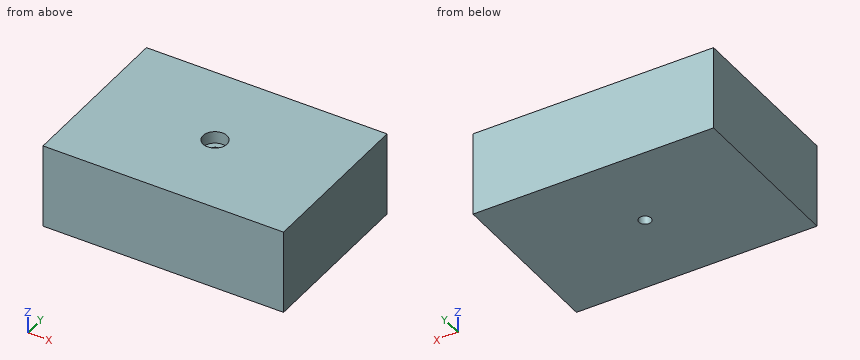
```python
from build123d import *

# Parameters (mm, degrees)
F0_W           = 100
F0_H           = 70
F1_DEPTH       = 17.5
F4_D           = 5
F4_CBORE_D     = 10
F4_CBORE_DEPTH = 5


with BuildPart() as f1:
    # F0 (on Top) → F1 (new body, symmetric)
    with BuildSketch(Plane.XY):
        Rectangle(F0_W, F0_H)
    extrude(amount=F1_DEPTH, both=True)

    # F4 (through all)
    with Locations(Plane.XY.offset(17.5)):
        with Locations((0, 0)):
            CounterBoreHole(F4_D / 2, F4_CBORE_D / 2, F4_CBORE_DEPTH)


solid = f1.part
```
The listing builds one solid part. Answer for the finished solid, in the listing's coordinates (mm). Coordinates: 2 decimals unless noted, no trailing zeros. Loops run counter-clockwise (first coordinate to the right, second up) from the corner with the lowest first, then second, coordinate; pieces in that order, holes last. Notation, with made-up numbers: (53, 88) -> (81, 88) arc R30 ccw to (81, 110) -> close; hole circle Ø5 at (47, -3.75). An arc over 180 degrees is marked (long way). Use one line per item in the form item = value. Start each with the question number.
Item 1: A flat-ended cylindrical pin translates along its axis: pin 1 Ø3 at (x, y) = (-2, 2) entering from +Z. Find the tip coordinate at first contact, or state that the pin passes through.
Item 2: Consider L1, parallel to Y at x = 0, z = 4; L2, parallel to Y at x = 0, z = 14.2; L3, parallel to X at y = 2, z = 9.5. Determine where each line is inside the solid, lowest interval first. Write a range as [from, to].
Item 3: The part is cut by section A-A on x = 0. Determine the outline of the cut face in (y, z).
Item 4: The part is cut by section B-B on y = 0. Determine the outline of the cut face in (x, z), then the cut area to 3 significant figures.
Answer key:
q1.pin_1 = 12.5
q2.L1 = [-35, -2.5], [2.5, 35]
q2.L2 = [-35, -5], [5, 35]
q2.L3 = [-50, -1.5], [1.5, 50]
q3.outline = (-35, -17.5) -> (-2.5, -17.5) -> (-2.5, 12.5) -> (-5, 12.5) -> (-5, 17.5) -> (-35, 17.5) -> close; (2.5, -17.5) -> (35, -17.5) -> (35, 17.5) -> (5, 17.5) -> (5, 12.5) -> (2.5, 12.5) -> close
q4.outline = (-50, -17.5) -> (-2.5, -17.5) -> (-2.5, 12.5) -> (-5, 12.5) -> (-5, 17.5) -> (-50, 17.5) -> close; (2.5, -17.5) -> (50, -17.5) -> (50, 17.5) -> (5, 17.5) -> (5, 12.5) -> (2.5, 12.5) -> close
q4.area = 3,300 mm2
